The figure shows three views and two pictorial views of one solid part (mm, origin at its lowest corner). Answer the questions. A direction names the side the tool comes from. Round coordinates to 2 decimals unless told otherwise and drop trailing zeros. Order: outer loops, then holes, each group sorted by start corner. A loop starts at its lowest first (then second) coordinate and runs counter-clockwise, first axis right, second up. Notation, with made-up numbers: (32.25, 55) - (58.25, 55) arc R13 ccw to (58.25, 63) - close; hole circle Ø3 at (-2, 55). An arc over 180 degrees is marked (long way). Use CSV: the item, a comma, the result in double quotes. Start each with the question number.
Item 1: Flat-ended cylindrical pins translate along their axes: P1, Ø1.3, axis at x = 25.5, z = 30.5, coming from the -Y side; P2, Ø12, axis at y = 14, z = 13.5, coming from the -X side; P3, Ø3, axis at x = 45, z = 30.5, coming from the -Y side; P4, Ø3, axis at y = 24, z = 5.5, coming from the -X side. Find the tip coordinate at first contact, or state that the pin passes through.
Item 2: Find section C-C, the plane x = 45. Give the vertices of the cut face in (y, z), plus the area to 3 significant figures.
Item 3: Straight lines are drawn through the part: line 1 along Z through (x, y) = (46, 24); line 2 along Z through (x, y) = (46, 5); line 3 along Z through (x, y) = (25, 16). For each, find the intervals that lie inside material, in ascending order. Write a range as [from, to].
Item 4: For the marked faces 1, 2, 3, 4 and 5, determine the directions among +Z, -Z, +X, -X, +Y, -Y from which every point of the face is accessible in a straight line to the end or side of a thin tool.
Item 5: Find section B-B, the plane y = 24. Give the vertices of the cut face in (x, z), plus the area to 3 significant figures.
Item 6: Find section A-A, the plane y = 14. Count the separate pieces of the cut face and the enclosed holes in it, plus the area to 3 significant figures.
Item 7: Find section D-D, the plane y = 6.5. Give the vertices of the cut face in (x, z), plus the area to 3 significant figures.
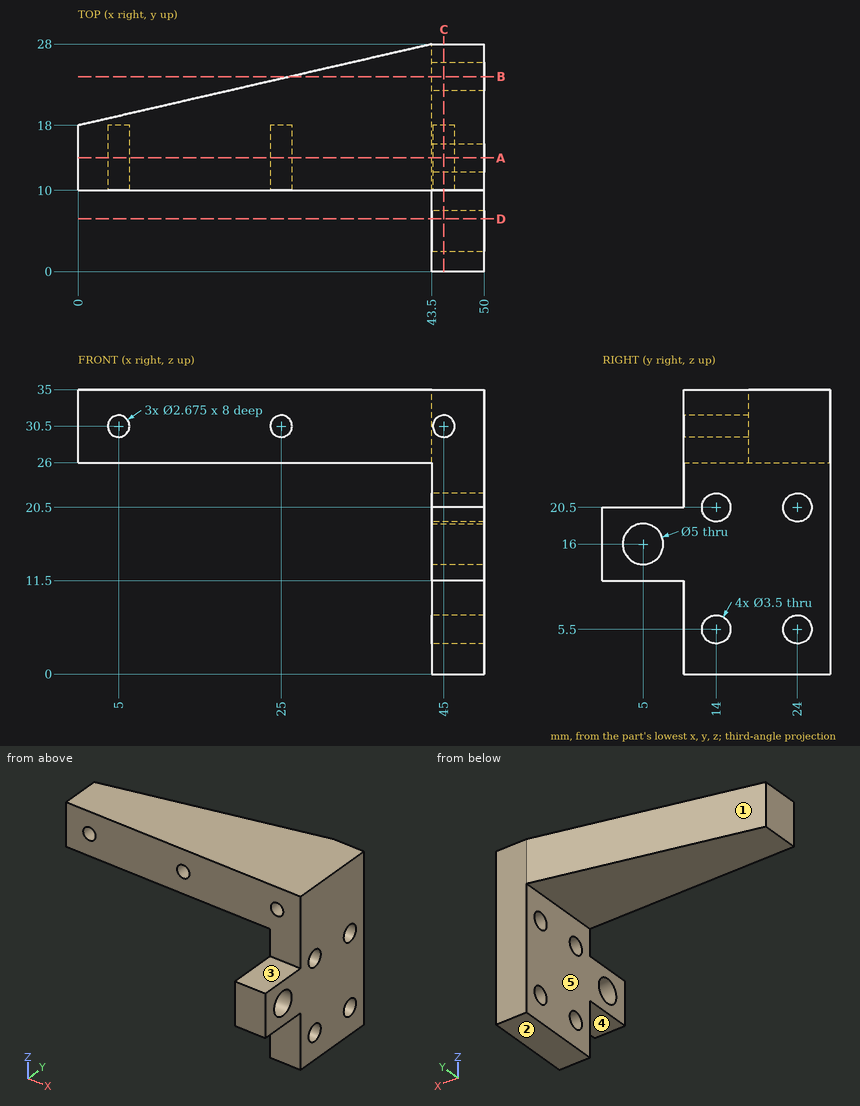
Worked out:
1,P1,"stops at y = 18"
1,P2,"stops at x = 43.5"
1,P3,"stops at y = 10"
1,P4,"passes through"
2,outline,"(0, 11.5) - (10, 11.5) - (10, 0) - (28, 0) - (28, 35) - (10, 35) - (10, 31.84) - (18, 31.84) - (18, 29.16) - (10, 29.16) - (10, 20.5) - (0, 20.5) - close; hole circle Ø5 at (5, 16); hole circle Ø3.5 at (14, 5.5); hole circle Ø3.5 at (14, 20.5); hole circle Ø3.5 at (24, 5.5); hole circle Ø3.5 at (24, 20.5)"
2,area,"640 mm²"
3,line 1,"z = [0, 3.75], [7.25, 18.75], [22.25, 35]"
3,line 2,"z = [11.5, 13.5], [18.5, 20.5]"
3,line 3,"z = [26, 29.16], [31.84, 35]"
4,face 1,"+Z, -Z, -X, +Y"
4,face 2,"-Z, +X, -X, +Y, -Y"
4,face 3,"+Z, +X, -X, -Y"
4,face 4,"-Z, +X, -X, -Y"
4,face 5,"-Z, -X, +Y, -Y"
5,outline,"(26.1, 26) - (43.5, 26) - (43.5, 22.25) - (50, 22.25) - (50, 35) - (26.1, 35) - close; (43.5, 0) - (50, 0) - (50, 3.75) - (43.5, 3.75) - close; (43.5, 7.25) - (50, 7.25) - (50, 18.75) - (43.5, 18.75) - close"
5,area,"339 mm²"
6,separate pieces,"3"
6,enclosed holes,"3"
6,area,"557 mm²"
7,outline,"(43.5, 11.5) - (50, 11.5) - (50, 14) - (43.5, 14) - close; (43.5, 18) - (50, 18) - (50, 20.5) - (43.5, 20.5) - close"
7,area,"32.5 mm²"
